```python
from build123d import *

# Parameters (mm, degrees)
F0_W     = 20
F0_H     = 20
F0_W_2   = 10.42
F0_H_2   = 10.42
F1_DEPTH = 1.6
F2_DEPTH = 12
F3_W     = 20
F3_H     = 20
F3_W_2   = 10.42
F3_H_2   = 10.42
F4_DEPTH = 1.6
F5_R     = 2


with BuildPart() as f1:
    # F0 (on Front) → F1 (new body)
    with BuildSketch(Plane.XZ):
        Rectangle(F0_W, F0_H)
        Rectangle(F0_W_2, F0_H_2, mode=Mode.SUBTRACT)
        Rectangle(F0_W_2, F0_H_2)
    extrude(amount=F1_DEPTH)

    # F0 (on Front) → F2 (join)
    with BuildSketch(Plane.XZ):
        Rectangle(F0_W, F0_H)
        Rectangle(F0_W_2, F0_H_2, mode=Mode.SUBTRACT)
    extrude(amount=F2_DEPTH)

    # F3 (on face) → F4 (join)
    with BuildSketch(Plane.XZ.offset(12)):
        Rectangle(F3_W, F3_H)
        Rectangle(F3_W_2, F3_H_2, mode=Mode.SUBTRACT)
        Rectangle(F3_W_2, F3_H_2)
    extrude(amount=F4_DEPTH)

    # F5
    f5_edges = [f1.edges().sort_by_distance(p)[0] for p in [
        (-10, -6.8, -10),
        (10, -6.8, -10),
        (10, -6.8, 10),
        (-10, -6.8, 10),
    ]]
    fillet(f5_edges, radius=F5_R)


solid = f1.part
```
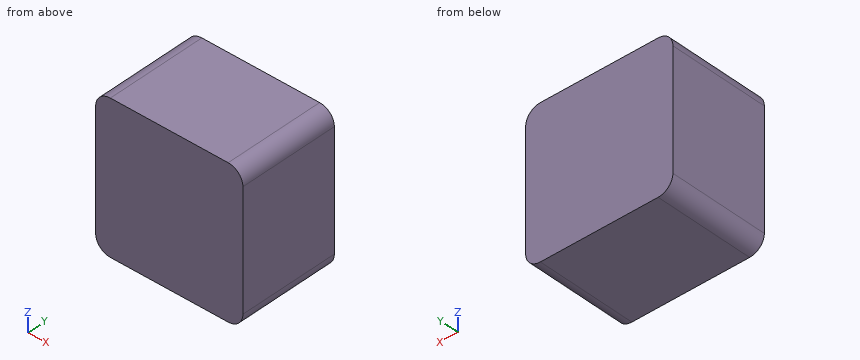
Model file for the job. Use its own axes, mm. Coordinates: 2 decimals unless noted, no trailing zeros. Order: outer loops, then holes, each group sorted by start corner. A loop starts at its lowest first (then second) coordinate and runs counter-clockwise, first axis right, second up. Notation, with made-up numbers: (48.5, 26) -> (66.5, 26) arc R22 ccw to (66.5, 41) -> close; hole circle Ø10 at (-16.75, 1). An arc over 180 degrees is marked (long way). Answer as a JSON object with one key per item and string values. Group by question number.
1) Cut at A-A, the plane y = -2. Write the cut outline in (x, z), then the cut area to 3 significant figures.
2) Drill centre lines: L1, parallel to X at y = -9.5, z = -1.75; L2, parallel to Y at x = -4.75, z = 4. Where is each one in solid material? Low to high.
3) Cut at B-B, the plane z = -3.25. Write the cut outline in (x, y).
Check values:
{
 "1": {"outline": "(-10, -8) arc R2 ccw to (-8, -10) -> (8, -10) arc R2 ccw to (10, -8) -> (10, 8) arc R2 ccw to (8, 10) -> (-8, 10) arc R2 ccw to (-10, 8) -> close; hole (-5.21, -5.21) -> (5.21, -5.21) -> (5.21, 5.21) -> (-5.21, 5.21) -> close", "area": "288 mm²"},
 "2": {"L1": "x = -10 to -5.21, 5.21 to 10", "L2": "y = -13.6 to -12, -1.6 to 0"},
 "3": {"outline": "(-10, -13.6) -> (10, -13.6) -> (10, 0) -> (-10, 0) -> close; hole (-5.21, -12) -> (5.21, -12) -> (5.21, -1.6) -> (-5.21, -1.6) -> close"}
}
